Verification items for this drawing (mm, ordinates from the low corner). Round coordinates to 2 decimals unless told otherwise and drop trailing zeros. Write each loop counter-clockwise with the first axis right and the second up, starting at its lowest first coordinate (ties: lowest second). Pieces come first, ordered by that corner, then holes. Notation, with made-up numbers: (38, 63) -> (51, 63) arc R20 cw to (51, 86) -> close; hole circle Ø1 at (36, -18). An arc over 180 degrees is marked (long way). Return JSON: item names as keys, results as strings. Group by question number.
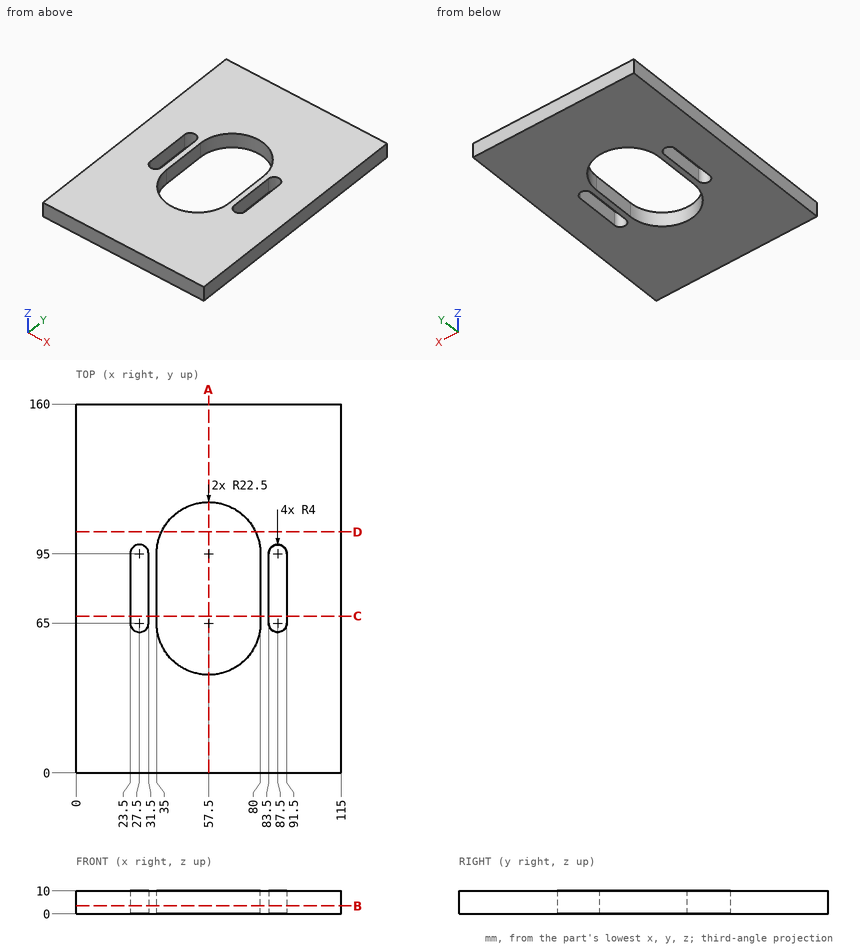
1) Material ranges on probe 1 along X at (y, z) = (86, 2.75); probe 2 along X at (y, z) = (63, 5.5); probe 3 along Y at (x, z) = (24, 2.25), recorded low to high. Write a range as [from, to].
2) Sectioned sample at D-D on y = 104.5. Enter the section's corners in (x, z), and give its area (3 significant figures).
3) Sectioned sample at C-C on y = 68. Enter the section's corners in (x, z).
4) Sectioned sample at A-A on x = 57.5. Enter the section's corners in (y, z).
5) Sectioned sample at B-B on z = 3.5. Enter the section's corners in (x, y), and give its area (3 significant figures).
Evaluation:
{
 "1": {"probe 1": "x = [0, 23.5], [31.5, 35], [80, 83.5], [91.5, 115]", "probe 2": "x = [0, 24.04], [30.96, 35.09], [79.91, 84.04], [90.96, 115]", "probe 3": "y = [0, 63.06], [96.94, 160]"},
 "2": {"outline": "(0, 0) -> (37.1, 0) -> (37.1, 10) -> (0, 10) -> close; (77.9, 0) -> (115, 0) -> (115, 10) -> (77.9, 10) -> close", "area": "742 mm2"},
 "3": {"outline": "(0, 0) -> (23.5, 0) -> (23.5, 10) -> (0, 10) -> close; (31.5, 0) -> (35, 0) -> (35, 10) -> (31.5, 10) -> close; (80, 0) -> (83.5, 0) -> (83.5, 10) -> (80, 10) -> close; (91.5, 0) -> (115, 0) -> (115, 10) -> (91.5, 10) -> close"},
 "4": {"outline": "(0, 0) -> (42.5, 0) -> (42.5, 10) -> (0, 10) -> close; (117.5, 0) -> (160, 0) -> (160, 10) -> (117.5, 10) -> close"},
 "5": {"outline": "(0, 0) -> (115, 0) -> (115, 160) -> (0, 160) -> close; hole (23.5, 65) arc R4 ccw to (31.5, 65) -> (31.5, 95) arc R4 ccw to (23.5, 95) -> close; hole (35, 65) arc R22.5 ccw to (80, 65) -> (80, 95) arc R22.5 ccw to (35, 95) -> close; hole (83.5, 65) arc R4 ccw to (91.5, 65) -> (91.5, 95) arc R4 ccw to (83.5, 95) -> close", "area": "14,900 mm2"}
}
